Can you work these out from the model? Positions are in its coordinate system, mm. A direction names the side the tool comes from. Round coordinates to 2 decimals unless told otherwise and drop trailing zeros. Loops run counter-clockwise (first coordinate to the right, second up) from the corner with the lowest first, then second, coordinate; pieces in that order, holes last. Notation, with made-up numbers: (-10, 37.5) -> (15, 37.5) arc R12 ccw to (15, 54.5) -> close; hole circle Ø4 at (-33.5, 82.25). An arc over 180 degrees is marked (long way). Answer as a JSON object with one key per item and string values.
```python
from build123d import *

# Parameters (mm, degrees)
SKETCH_1_R      = 25
EXTRUDE_1_DEPTH = 5
SKETCH_2_R      = 20
EXTRUDE_2_DEPTH = 5
SKETCH_3_R      = 15
EXTRUDE_3_DEPTH = 5
SKETCH_4_R      = 10
EXTRUDE_4_DEPTH = 5


with BuildPart() as part:
    # Эскиз1 → Бобышка-Вытянуть1 (new body)
    with BuildSketch(Plane.XY):
        Circle(SKETCH_1_R)
    extrude(amount=EXTRUDE_1_DEPTH)

    # Эскиз2 → Бобышка-Вытянуть2 (add)
    with BuildSketch(Plane.XY.offset(5)):
        Circle(SKETCH_2_R)
    extrude(amount=EXTRUDE_2_DEPTH)

    # Эскиз3 → Бобышка-Вытянуть3 (add)
    with BuildSketch(Plane.XY.offset(10)):
        Circle(SKETCH_3_R)
    extrude(amount=EXTRUDE_3_DEPTH)

    # Эскиз4 → Бобышка-Вытянуть4 (add)
    with BuildSketch(Plane.XY.offset(15)):
        Circle(SKETCH_4_R)
    extrude(amount=EXTRUDE_4_DEPTH)


solid = part.part
```
Q1. If I drill on L1, parallel to Z at x = 14, y = -16; L2, parallel to Z at x = 6.5, y = 14.5; L3, parallel to X at y = 0.5, z = 15.75, over which ranges is the centre line in solid material (lowest first)? Write a range as [from, to].
Determined:
{"L1": "[0, 5]", "L2": "[0, 10]", "L3": "[-9.99, 9.99]"}
Q2. I want a section at C-C, the plane z = 13.25. Write out the boundary of the cut face in (x, y).
Determined:
{"outline": "circle Ø30 at (0, 0)"}
Q3. I want a section at A-A, the plane x = 0. Write out the boundary of the cut face in (y, z).
Determined:
{"outline": "(-25, 0) -> (25, 0) -> (25, 5) -> (20, 5) -> (20, 10) -> (15, 10) -> (15, 15) -> (10, 15) -> (10, 20) -> (-10, 20) -> (-10, 15) -> (-15, 15) -> (-15, 10) -> (-20, 10) -> (-20, 5) -> (-25, 5) -> close"}
Q4. We'd pull the mould along X, two halves only. Please class faces 3 (the cylindrical face through (-14.985, 0.66, 12.465)), 4 (the flat face through (3, 15, 10)): pulls with the +X half, pulls with the -X half, needs draft (parallel to the pull), parting line crosses it, or undercut.
Determined:
{"face 3": "parting line crosses it", "face 4": "needs draft"}
Q5. On a 3-axis mill with a long thin cutter (end or side, diameter ignored), from which of +Z, -Z, +X, -X, +Y, -Y can I reach the whole of each face in a straight line? I mean faces 1 (the cylindrical face through (-2.17, -9.76, 17.46)), 2 (the flat face through (0, 0, 20)). Say none if no direction works.
Determined:
{"face 1": "+Z", "face 2": "+Z, +X, -X, +Y, -Y"}
Q6. I want a section at D-D, the plane y = 17. Write out the boundary of the cut face in (x, z), then the cut area to 3 significant figures.
Determined:
{"outline": "(-18.33, 0) -> (18.33, 0) -> (18.33, 5) -> (10.54, 5) -> (10.54, 10) -> (-10.54, 10) -> (-10.54, 5) -> (-18.33, 5) -> close", "area": "289 mm²"}
Q7. I'm going to push flat-ended pins straight in: pin 1 (5 mm diameter, centred on x = -13.5, y = -2, fed in from +Z); pin 2 (10 mm diameter, centred on y = -5.5, z = 5, fed in from -X) (3 decimals); pin 3 (6 mm diameter, centred on y = 8, z = 2.5, fed in from -X); pin 4 (1 mm diameter, centred on y = 11.5, z = 16, fed in from +X). Where does each tip first touch, or does it pass through?
Determined:
{"pin 1": "z = 15", "pin 2": "x = -24.995", "pin 3": "x = -24.49", "pin 4": "through"}
